The listing builds one solid part. Answer for the finished solid, in the listing's coordinates (mm). A direction names the side the tool comes from. Coordinates: 2 decimals unless noted, no trailing zeros. Write each loop counter-clockwise with the first axis right and the second up, starting at its lowest first coordinate (ties: lowest second). Pieces come first, ordered by that corner, then holes.
from build123d import *

# Parameters (mm, degrees)
SKETCH_W     = 101.6
SKETCH_H     = 101.6
PAD_DEPTH    = 304.8
FILLET_R     = 19.05
SKETCH001_W  = 88.9
SKETCH001_H  = 88.9
POCKET_DEPTH = 304.801
FILLET001_R  = 12.7


with BuildPart() as part:
    # Sketch → Pad (new body)
    with BuildSketch(Plane.YZ):
        Rectangle(SKETCH_W, SKETCH_H)
    extrude(amount=PAD_DEPTH)

    # Fillet
    fillet_edges = [part.edges().sort_by_distance(p)[0] for p in [
        (152.4, 50.8, 50.8),
        (152.4, -50.8, 50.8),
        (152.4, 50.8, -50.8),
        (152.4, -50.8, -50.8),
    ]]
    fillet(fillet_edges, radius=FILLET_R)

    # Sketch001 → Pocket (cut, through all)
    with BuildSketch(Plane.YZ):
        Rectangle(SKETCH001_W, SKETCH001_H)
    extrude(amount=POCKET_DEPTH, mode=Mode.SUBTRACT)

    # Fillet001
    fillet001_edges = [part.edges().sort_by_distance(p)[0] for p in [
        (152.4, -44.45, -44.45),
        (152.4, -44.45, 44.45),
        (152.4, 44.45, 44.45),
        (152.4, 44.45, -44.45),
    ]]
    fillet(fillet001_edges, radius=FILLET001_R)


solid = part.part
1. A tool of negligible diameter and unlimited length cuts with its end or side. For faces 5 (the flat face through (150, -44.45, 0)), 6 (the cylindrical face through (154.53, 45.07, -45.37)), from which of +Z, -Z, +X, -X, +Y, -Y can it reach the whole face along a straight path? Write none if from no direction.
Results found:
face 5: +X, -X
face 6: -Z, +X, -X, +Y
2. Section A-A on y = -6 is taken. Give the vertices of the cut face in (x, z).
Results found:
outline: (0, -50.8) - (304.8, -50.8) - (304.8, -44.45) - (0, -44.45) - close; (0, 44.45) - (304.8, 44.45) - (304.8, 50.8) - (0, 50.8) - close
3. Section C-C on x = 194 is taken. Give the vertices of the cut face in (y, z).
Results found:
outline: (-50.8, -31.75) arc R19.05 ccw to (-31.75, -50.8) - (31.75, -50.8) arc R19.05 ccw to (50.8, -31.75) - (50.8, 31.75) arc R19.05 ccw to (31.75, 50.8) - (-31.75, 50.8) arc R19.05 ccw to (-50.8, 31.75) - close; hole (-44.45, -31.75) arc R12.7 ccw to (-31.75, -44.45) - (31.75, -44.45) arc R12.7 ccw to (44.45, -31.75) - (44.45, 31.75) arc R12.7 ccw to (31.75, 44.45) - (-31.75, 44.45) arc R12.7 ccw to (-44.45, 31.75) - close
4. For a pull along Y with two mould halves and no side action, classify faces 1 (the flat face through (150, 0, -44.45)), 2 (the cylindrical face through (154.53, 40.63, -40.83)), 3 (the flat face through (150, -50.8, 0)), 4 (the cylindrical face through (154.53, 45.37, 45.07)) as pulls with the +Y half, pulls with the -Y half, needs draft (parallel to the pull), parting line crosses it, or undercut.
Results found:
face 1: undercut
face 2: undercut
face 3: pulls with the -Y half
face 4: pulls with the +Y half
5. Find the intervals of material crossed by L1, parallel to Y at x = 22.5, z = 25; L2, parallel to Y at x = 230, z = -46, in increasing order.
Results found:
L1: y = -50.8 to -44.45, 44.45 to 50.8
L2: y = -44.39 to 44.39
